Model file for the job. Use its own axes, mm. Coordinates: 2 decimals unless noted, no trailing zeros. Write each loop counter-clockwise with the first axis right and the second up, starting at its lowest first coordinate (ties: lowest second). Pieces come first, ordered by that corner, then holes. Notation, with made-up numbers: M 28,-11.75 L 50,-11.75 A19 ccw 50,13.25 Z; hole C -12,42.25 d11. An arc over 180 degrees is marked long. One line per question, with ' | ' between items. Start each with the question number.
(1) Cut at C-C (y = 0.65). Count the separate pieces of the cut face and the enclosed holes in it, plus the area to 3 significant figures.
(2) Cut at D-D (z = -32.5). Write the cut outline in (x, y), plus the area to 3 significant figures.
(3) Cut at A-A (z = -18). Write the cut outline in (x, y), plus the area to 3 significant figures.
(4) Flat gauge pins, fed straight in: pin 1 Ø0.6 at (y, z) = (1, -27.5) entering from -X; pin 2 Ø1 at (x, y) = (-29, 0.5) entering from -Z; pin 3 Ø0.6 at (y, z) = (1, 17) entering from +X. Where does each tip first touch, or does it go through?
(5) Cut at B-B (x = -5). Write the cut outline in (y, z), plus the area to 3 significant figures.
(6) Wall check: probe 1 along X at (y, z) = (0.6, -3); probe 2 along Z at (x, y) = (-4, 1); probe 3 along X at (y, z) = (1.5, 8.5). Give the ranges that are in metal, low to high.
Autodesk Inventor part; units mm, degrees
ref_plane "YZ Plane" through (0, 0, 0) normal (1, 0, 0) x (0, 1, 0)
ref_plane "XZ Plane" through (0, 0, 0) normal (0, 1, 0) x (-1, 0, 0)
ref_plane "XY Plane" through (0, 0, 0) normal (0, 0, 1) x (1, 0, 0)
sketch "Sketch1" plane through (0, 0, 0) normal (0, 1, 0) x (-1, 0, 0)
  point P0 (0, 0)
sketch "Sketch2" plane through (0, 0, 0) normal (0, 1, 0) x (-1, 0, 0)
  line L0 (55.6, -39.5) -> (55.6, -37.5)
  line L1 (55.6, -39.5) -> (37.3, -39.5)
  line L2 (37.3, -39.5) -> (37.3, -37.5)
  line L3 (37.3, -37.5) -> (19, -37.5)
  line L4 (19, -37.5) -> (19, -39.5)
  line L5 (19, -39.5) -> (0.7, -39.5)
  line L6 (-1.34, -37.5) -> (-17.6, -37.5)
  line L7 (-17.6, -37.5) -> (-17.6, -39.5)
  line L8 (-17.6, -39.5) -> (-35.9, -39.5)
  line L9 (-35.9, -39.5) -> (-35.9, -37.5)
  line L10 (-35.9, -37.5) -> (-53, -37.5)
  line L11 (-55, 37.5) -> (-36.7, 37.5)
  line L12 (-18.4, 37.5) -> (-0.1, 37.5)
  line L13 (18.2, 37.5) -> (36.5, 37.5)
  line L14 (55.6, 35.5) -> (55.6, 25)
  line L15 (55.6, 12.5) -> (55.6, 0)
  line L16 (55.6, -12.5) -> (55.6, -25)
  line L17 (55.6, 25) -> (53.6, 25)
  line L18 (53.6, 25) -> (53.6, 12.5)
  line L19 (53.6, 12.5) -> (55.6, 12.5)
  line L20 (55.6, 0) -> (53.6, 0)
  line L21 (53.6, 0) -> (53.6, -12.5)
  line L22 (53.6, -12.5) -> (55.6, -12.5)
  line L23 (55.6, -25) -> (53.6, -25)
  line L24 (53.6, -25) -> (53.6, -37.5)
  line L25 (53.6, -37.5) -> (55.6, -37.5)
  line L26 (36.5, 37.5) -> (36.5, 35.5)
  line L27 (36.5, 35.5) -> (55.6, 35.5)
  line L28 (18.2, 37.5) -> (18.2, 35.5)
  line L29 (18.2, 35.5) -> (-0.1, 35.5)
  line L30 (-0.1, 35.5) -> (-0.1, 37.5)
  line L31 (-18.4, 37.5) -> (-18.4, 35.5)
  line L32 (-18.4, 35.5) -> (-36.7, 35.5)
  line L33 (-36.7, 35.5) -> (-36.7, 37.5)
  line L34 (37.75, -22.5) -> (35.25, -22.5)
  line L35 (35.25, -22.5) -> (35.25, 22.5)
  line L36 (35.25, 22.5) -> (37.75, 22.5)
  line L37 (37.75, 22.5) -> (37.75, -22.5)
  line L38 (37.75, -22.5) -> (35.25, 22.5) construction
  line L39 (35.25, -22.5) -> (37.75, 22.5) construction
  line L40 (-37.75, -22.5) -> (-35.25, -22.5)
  line L41 (-35.25, -22.5) -> (-35.25, 22.5)
  line L42 (-35.25, 22.5) -> (-37.75, 22.5)
  line L43 (-37.75, 22.5) -> (-37.75, -22.5)
  line L44 (-37.75, -22.5) -> (-35.25, 22.5) construction
  line L45 (-35.25, -22.5) -> (-37.75, 22.5) construction
  line L46 (15, -28.4801) -> (-15, -28.4801)
  line L47 (-15, -28.4801) -> (-15, -25.9801)
  line L48 (-15, -25.9801) -> (15, -25.9801)
  line L49 (15, -25.9801) -> (15, -28.4801)
  line L50 (15, -28.4801) -> (-15, -25.9801) construction
  line L51 (-15, -28.4801) -> (15, -25.9801) construction
  line L52 (15, 28.4801) -> (-15, 28.4801)
  line L53 (-15, 28.4801) -> (-15, 25.9801)
  line L54 (-15, 25.9801) -> (15, 25.9801)
  line L55 (15, 25.9801) -> (15, 28.4801)
  line L56 (15, 28.4801) -> (-15, 25.9801) construction
  line L57 (-15, 28.4801) -> (15, 25.9801) construction
  line L58 (-53, -37.5) -> (-55, -37.5)
  line L59 (-57, -22.5) -> (-57, -22.4801)
  line L60 (-57, 37.5) -> (-55, 37.5)
  line L61 (-55, -37.5) -> (-57, -37.5)
  line L62 (-57, -37.5) -> (-57, -25)
  line L63 (-57, -25) -> (-59.4283, -25)
  line L64 (-59.4283, -25) -> (-59.4283, -12.5)
  line L65 (-59.4283, -12.5) -> (-57, -12.5)
  line L66 (-57, 0) -> (-57, -12.5)
  line L67 (-57, 0) -> (-59, 0)
  line L68 (-59, 0) -> (-59, 12.5)
  line L69 (-59, 12.5) -> (-57, 12.5)
  line L70 (-57, 12.5) -> (-57, 25)
  line L71 (-57, 25) -> (-59.4283, 25)
  line L72 (-59.4283, 25) -> (-59.4283, 37.5)
  line L73 (-59.4283, 37.5) -> (-57, 37.5)
  line L74 (0.7, -39.5) -> (-1.34, -39.5)
  line L75 (-1.34, -39.5) -> (-1.34, -37.5)
  point P0 (0.7, -37.5)
  point P1 (-55, 22.5)
  point P2 (-53, 22.5)
  point P3 (-53, 0)
  point P4 (-53, -12.5)
  point P5 (36.5, 0)
  point P6 (-36.5, 0)
  point P7 (0, -27.2301)
  point P8 (0, 27.2301)
  dimension "d55" = 18.3
  dimension "d56" = 2.04
extrude "Extrusion1" add sketch "Sketch2" along normal blind 2
properties part number "BLKG"
Filled in:
1) separate pieces: 1 | enclosed holes: 4 | area: 8,080 mm²
2) outline: M -53.6,0 L 57,0 L 57,2 L -53.6,2 Z | area: 221 mm²
3) outline: M -55.6,0 L -37.75,0 L -37.75,2 L -55.6,2 Z; M -35.25,0 L 35.25,0 L 35.25,2 L -35.25,2 Z; M 37.75,0 L 59.43,0 L 59.43,2 L 37.75,2 Z | area: 220 mm²
4) pin 1: x = -53.6 | pin 2: z = -37.5 | pin 3: x = 57
5) outline: M 0,-39.5 L 2,-39.5 L 2,-28.48 L 0,-28.48 Z; M 0,-25.98 L 2,-25.98 L 2,25.98 L 0,25.98 Z; M 0,28.48 L 2,28.48 L 2,35.5 L 0,35.5 Z | area: 140 mm²
6) probe 1: -53.6 to -37.75, -35.25 to 35.25, 37.75 to 57 | probe 2: -39.5 to -28.48, -25.98 to 25.98, 28.48 to 35.5 | probe 3: -55.6 to -37.75, -35.25 to 35.25, 37.75 to 59
